Here's the drawing with two shaded views (mm, measured from the low corner). I have some questions. Coordinates: 2 decimals unless noted, no trailing zeros. Write each loop counter-clockwise with the first axis right and the second up, starting at its lowest first coordinate (ties: lowest second). Pieces come first, ordered by that corner, then holes. Notation, with made-up numbers: (30, 66.5) -> (70, 66.5) arc R15 cw to (70, 93.5) -> close; hole circle Ø1 at (46.25, 3.5). An arc over 180 degrees is marked (long way). Use one line per item in the form item = value.
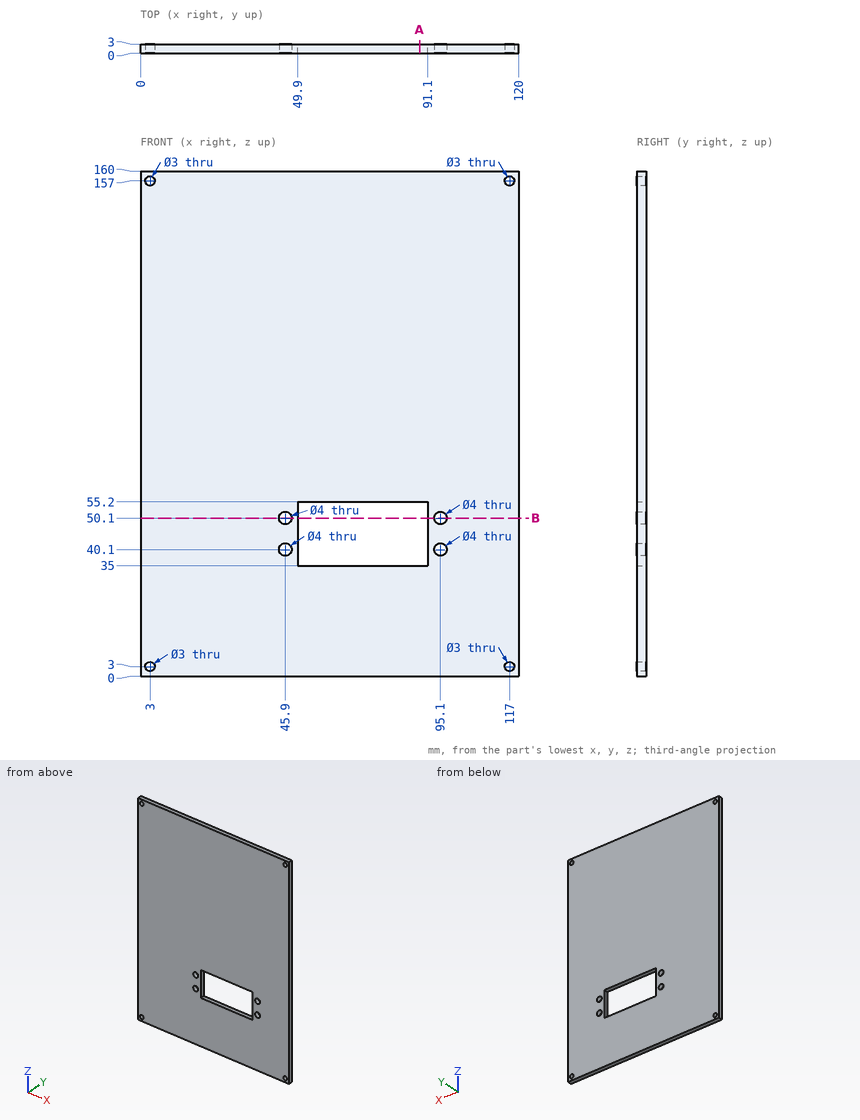
Q1. Suppose I cut it at B-B (z = 50.1). Write out the boundary of the cut face in (x, y).
Return value:
outline = (0, 0) -> (43.9, 0) -> (43.9, 3) -> (0, 3) -> close; (47.9, 0) -> (49.9, 0) -> (49.9, 3) -> (47.9, 3) -> close; (91.1, 0) -> (93.1, 0) -> (93.1, 3) -> (91.1, 3) -> close; (97.1, 0) -> (120, 0) -> (120, 3) -> (97.1, 3) -> close
Q2. Will this pin go through, and if not, where does the flat tip stop? pin 1 (2.5 mm diameter, centred on x = 3, z = 157, fed in from -Y).
Return value:
pin_1 = through
Q3. If I drill on line 1 (X direction, y = 1.15, z = 40.1); line 2 (X direction, y = 0.75, z = 157); line 3 (Z direction, x = 62, y = 0.5), over which ranges is the centre line in solid material (lowest first)? Write a range as from..to.
Return value:
line_1 = 0..43.9, 47.9..49.9, 91.1..93.1, 97.1..120
line_2 = 0..1.5, 4.5..115.5, 118.5..120
line_3 = 0..35, 55.2..160
Q4. Suppose I cut it at A-A (x = 88.5). Write out the boundary of the cut face in (y, z).
Return value:
outline = (0, 0) -> (3, 0) -> (3, 35) -> (0, 35) -> close; (0, 55.2) -> (3, 55.2) -> (3, 160) -> (0, 160) -> close
